Source: CAD feature listing. Evaluate the final solid. Frame: model axes, mm. Give positions to 0.01 mm unless a question says otherwise; leave off trailing zeros. Write each loop counter-clockwise with the first axis right and the second up, starting at its lowest first coordinate (ties: lowest second). Pieces come first, ordered by that corner, then holes. Notation, with made-up numbers: (89.25, -17.75) -> (101.25, -17.75) arc R19 cw to (101.25, 17.25) -> close; hole circle Ø5 at (41.25, -24.5). An arc over 180 degrees is marked (long way). Write item = value, one per line.
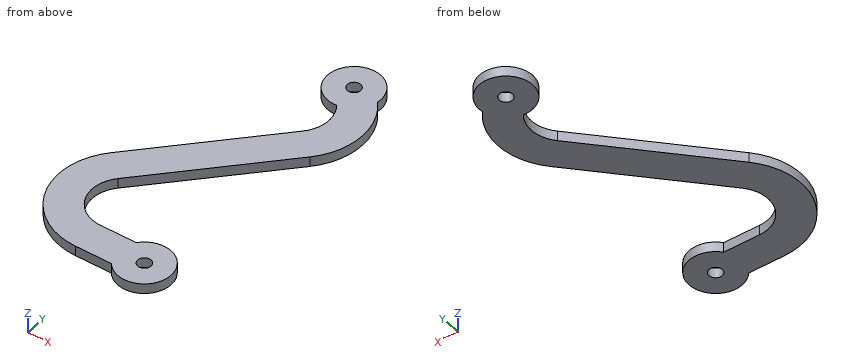
from build123d import *

# Parameters (mm, degrees)
SKETCH1_R           = 1
BOSS_EXTRUDE1_DEPTH = 1.5


with BuildPart() as part:
    # Sketch1 → Boss-Extrude1 (new body)
    with BuildSketch(Plane.XY):
        with BuildLine():
            Line((-3.122498999, 2.5), (-8.582047484, 2.5))
            ThreePointArc((-8.582047484, 2.5), (-13.162149565, 5.494341772), (-12.256495253, 10.89093403))
            Line((-12.256495253, 10.89093403), (3.737859555, 28.222566206))
            ThreePointArc((3.737859555, 28.222566206), (6.38742077, 34.828756828), (3.971570907, 41.523949028))
            ThreePointArc((3.971570907, 41.523949028), (-2.793624676, 44.86280652), (0.378773293, 38.017974034))
            ThreePointArc((0.378773293, 38.017974034), (1.382913373, 34.75852813), (0.063411786, 31.613500235))
            Line((0.063411786, 31.613500235), (-15.930943021, 14.281868059))
            ThreePointArc((-15.930943021, 14.281868059), (-17.742251646, 3.488683545), (-8.582047484, -2.5))
            Line((-8.582047484, -2.5), (-3.122498999, -2.5))
            ThreePointArc((-3.122498999, -2.5), (4, 0), (-3.122498999, 2.5))
        make_face()
        Circle(SKETCH1_R, mode=Mode.SUBTRACT)
        with Locations((0, 42)):
            Circle(SKETCH1_R, mode=Mode.SUBTRACT)
    extrude(amount=BOSS_EXTRUDE1_DEPTH)


solid = part.part
1) Material intervals for L1, parallel to Y at x = 0, z = 1.2; L2, parallel to Y at x = -2.75, z = 0.85; L3, parallel to Y at x = -11, z = 0.8, sorted ascending.
Computed:
L1 = -4 to -1, 1 to 4, 24.17 to 31.54, 38 to 41, 43 to 46
L2 = -2.9 to 2.9, 21.19 to 28.56, 39.1 to 44.9
L3 = -2.2 to 3.12, 12.25 to 19.63
2) Cut plane B-B (x = -0.5). Return the cut outline in (y, z), then the cut area to 3 significant figures.
Computed:
outline = (-3.97, 0) -> (-0.87, 0) -> (-0.87, 1.5) -> (-3.97, 1.5) -> close; (0.87, 0) -> (3.97, 0) -> (3.97, 1.5) -> (0.87, 1.5) -> close; (23.63, 0) -> (31, 0) -> (31, 1.5) -> (23.63, 1.5) -> close; (38.03, 0) -> (41.13, 0) -> (41.13, 1.5) -> (38.03, 1.5) -> close; (42.87, 0) -> (45.97, 0) -> (45.97, 1.5) -> (42.87, 1.5) -> close
area = 29.7 mm²
3) Cut plane A-A (y = 42). Return the cut outline in (x, z).
Computed:
outline = (-4, 0) -> (-1, 0) -> (-1, 1.5) -> (-4, 1.5) -> close; (1, 0) -> (4, 0) -> (4, 1.5) -> (1, 1.5) -> close
4) Contact query for a flat-ended pin moving along its axis: pin 1 (1.6 mm diameter, centred on x = 0, y = 0, fed in from -Z). Output: stop coordinate, or through.
Computed:
pin_1 = through
5) Cut plane D-D (x = -9.5). Return the cut outline in (y, z).
Computed:
outline = (-2.46, 0) -> (2.58, 0) -> (2.58, 1.5) -> (-2.46, 1.5) -> close; (13.88, 0) -> (21.25, 0) -> (21.25, 1.5) -> (13.88, 1.5) -> close
6) Cut plane C-C (z = 0.65). Return the cut outline in (x, y), then the cut area to 3 significant figures.
Computed:
outline = (-15.93, 14.28) arc R10 ccw to (-8.58, -2.5) -> (-3.12, -2.5) arc R4 ccw (long way) to (-3.12, 2.5) -> (-8.58, 2.5) arc R5 cw to (-12.26, 10.89) -> (3.74, 28.22) arc R10 ccw to (3.97, 41.52) arc R4 ccw (long way) to (0.38, 38.02) arc R5 cw to (0.06, 31.61) -> close; hole circle Ø2 at (0, 0); hole circle Ø2 at (0, 42)
area = 374 mm²
